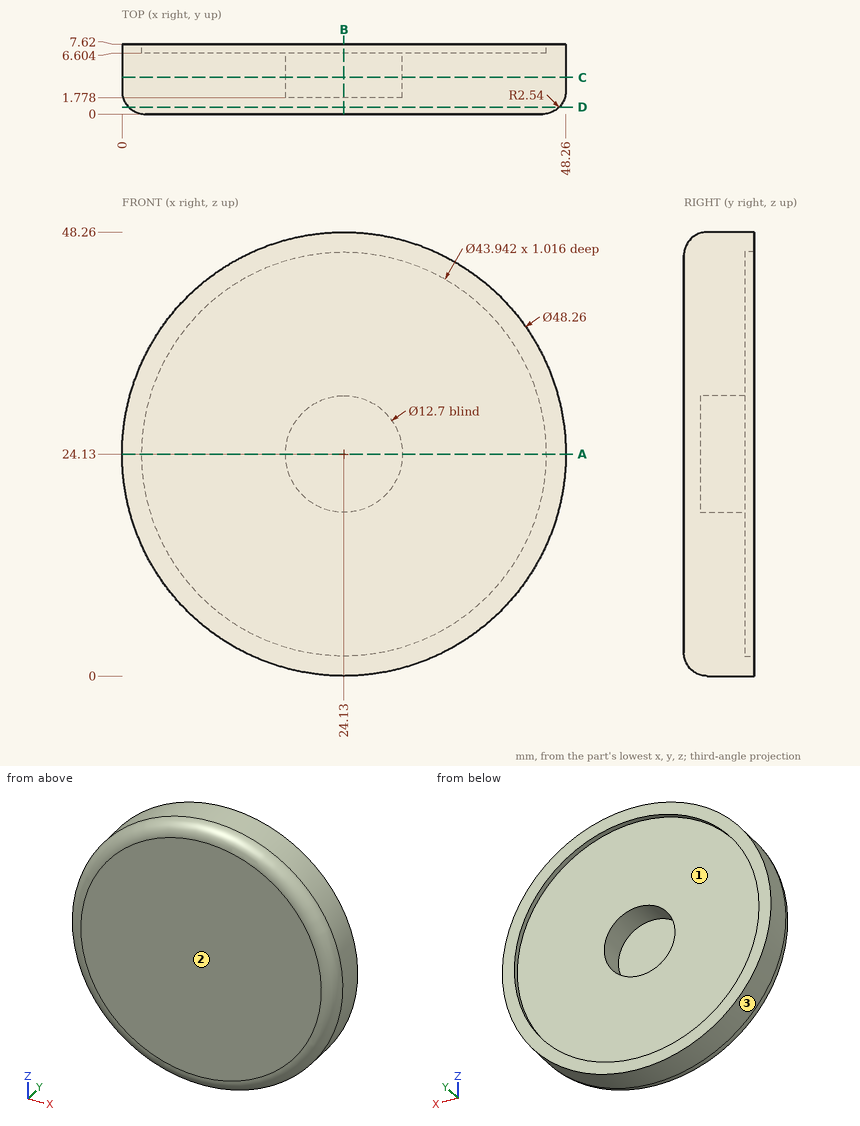
The drawing under review shows one solid part. Ordinate dimensions are in mm from its lowest x, y, z. Round coordinates to 2 decimals unless told otherwise and drop trailing zeros. Loops run counter-clockwise (first coordinate to the right, second up) from the corner with the lowest first, then second, coordinate; pieces in that order, holes last. Notation, with made-up numbers: M 36,22.5 L 75,22.5 A17 cw 75,36.5 Z; hole C 59,75 d9. An arc over 180 degrees is marked long. Answer as CSV lines item,"result". Start each with the question number.
Item 1: Consider section D-D (y = 0.75). Write out the cut boundary in (x, z).
Item 2: Consider section C-C (y = 4). Write out the cut boundary in (x, z), then the cut area to 3 significant figures.
Item 3: Mouldability with a two-part tool opening along Z and no side actions: class the marked faces 1, 2 and 3 as released by +Z, released by -Z, zero draft, split by the parting line, or undercut.
Item 4: Consider section B-B (x = 24.13). Write out the cut boundary in (y, z), then the cut area to 3 significant figures.
Item 5: Insertion check: P1, Ø4, axis at x = 21, z = 42, coming from the +Y side; P2, Ø2, axis at y = 2.5, z = 5.5, coming from the -X side; P3, Ø1.5, axis at x = 30, y = 5, coming from the -Z side. Each pin has a flat end and moves straight along its axis. Give the tip position at first contact, or say it passes through.
Item 6: Consider section A-A (z = 24.13). Write out the cut boundary in (x, y), then the cut area to 3 significant figures.
Item 7: Wall thickness on line 1 (X direction, y = 7.25, z = 24.13); line 2 (X direction, y = 2.85, z = 24.13); line 3 (Y direction, x = 41.5, z = 23): over which ranges is each line inside the solid? List them lowest first. Write a range as [from, to].
Answer:
1,outline,"C 24.13,24.13 d46.78"
2,outline,"C 24.13,24.13 d48.26; hole C 24.13,24.13 d12.7"
2,area,"1,700 mm^2"
3,face 1,"undercut"
3,face 2,"zero draft"
3,face 3,"split by the parting line"
4,outline,"M 0,2.54 A2.54 ccw 2.54,0 L 7.62,0 L 7.62,2.16 L 6.6,2.16 L 6.6,17.78 L 1.78,17.78 L 1.78,30.48 L 6.6,30.48 L 6.6,46.1 L 7.62,46.1 L 7.62,48.26 L 2.54,48.26 A2.54 ccw 0,45.72 Z"
4,area,"259 mm^2"
5,P1,"stops at y = 6.6"
5,P2,"stops at x = 7.65"
5,P3,"stops at z = 0.55"
6,outline,"M 0,2.54 A2.54 ccw 2.54,0 L 45.72,0 A2.54 ccw 48.26,2.54 L 48.26,7.62 L 46.1,7.62 L 46.1,6.6 L 30.48,6.6 L 30.48,1.78 L 17.78,1.78 L 17.78,6.6 L 2.16,6.6 L 2.16,7.62 L 0,7.62 Z"
6,area,"259 mm^2"
7,line 1,"x = [0, 2.16], [46.1, 48.26]"
7,line 2,"x = [0, 17.78], [30.48, 48.26]"
7,line 3,"y = [0, 6.6]"
